```python
from build123d import *

# Parameters (mm, degrees)
F1_DEPTH = 25.4
F3_D     = 12.7
F4_D     = 12.7
F5_R     = 5.08


with BuildPart() as f1:
    # F0 (on Front) → F1 (new body)
    with BuildSketch(Plane.XZ):
        with BuildLine():
            Line((-25.4, 19.05), (-50.8, 19.05))
            Line((-50.8, 19.05), (-50.8, -19.05))
            Line((-50.8, -19.05), (50.8, -19.05))
            Line((50.8, -19.05), (50.8, 19.05))
            Line((50.8, 19.05), (25.4, 19.05))
            ThreePointArc((25.4, 19.05), (0, -6.35), (-25.4, 19.05))
        make_face()
    extrude(amount=F1_DEPTH)

    # F3 (through all)
    with Locations(Plane.XY.offset(19.05)):
        with Locations((-38.1, -12.7)):
            Hole(F3_D / 2)

    # F4 (through all)
    with Locations(Plane.XY.offset(19.05)):
        with Locations((38.1, -12.7)):
            Hole(F4_D / 2)

    # F5
    f5_edges = [f1.edges().sort_by_distance(p)[0] for p in [
        (50.8, 0, 0),
        (-50.8, 0, 0),
        (0, 0, -19.05),
        (-50.8, -12.7, -19.05),
        (-50.8, -12.7, 19.05),
        (-50.8, -25.4, 0),
        (0, -25.4, -19.05),
        (50.8, -25.4, 0),
    ]]
    fillet(f5_edges, radius=F5_R)


solid = f1.part
```
The listing builds one solid part. Answer for the finished solid, in the listing's coordinates (mm). Give positions to 0.01 mm unless a question says otherwise; leave off trailing zeros. Order: outer loops, then holes, each group sorted by start corner. A loop starts at its lowest first (then second) coordinate and runs counter-clockwise, first axis right, second up. Notation, with made-up numbers: (35, -5.5) -> (93, -5.5) arc R29 ccw to (93, 22.5) -> close; hole circle Ø10 at (54, 28.5). An arc over 180 degrees is marked (long way). One line per item, written item: value.
1) A flat-ended cylindrical pin translates along its axis: P1, Ø3, axis at x = 3.5, y = -11.5, coming from the +Z side. Find the tip coordinate at first contact, or state that the pin passes through.
Reported:
P1: stops at z = -5.85
2) Determine the mould class of faces 1 (the cylindrical face through (32.234, -15.132, -0.267)), 2 (the flat face through (-50.8, -13, 0)), 3 (the cylindrical face through (-31.756, -12.421, -0.267)), 4 (the flat face through (2, -13, -19.05)) for opening direction X: pulls with the +X half, pulls with the -X half, needs draft (parallel to the pull), parting line crosses it, or undercut.
Reported:
face 1: undercut
face 2: pulls with the -X half
face 3: undercut
face 4: needs draft
3) Find section B-B, the plane y = -12.7. Determine the outline of the cut face in (x, z).
Reported:
outline: (-50.8, -13.97) arc R5.08 ccw to (-45.72, -19.05) -> (-44.45, -19.05) -> (-44.45, 19.05) -> (-45.72, 19.05) arc R5.08 ccw to (-50.8, 13.97) -> close; (-31.75, -19.05) -> (31.75, -19.05) -> (31.75, 19.05) -> (25.4, 19.05) arc R25.4 cw to (-25.4, 19.05) -> (-31.75, 19.05) -> close; (44.45, -19.05) -> (50.8, -19.05) -> (50.8, 19.05) -> (44.45, 19.05) -> close
4) Find section D-D, the plane z = 15.5. Determine the outline of the cut face in (x, y).
Reported:
outline: (-50.56, -21.85) arc R5.08 ccw to (-45.72, -25.4) -> (-25.15, -25.4) -> (-25.15, 0) -> (-45.72, 0) arc R5.08 ccw to (-50.56, -3.55) -> close; (25.15, -25.4) -> (45.72, -25.4) arc R5.08 ccw to (50.8, -20.32) -> (50.8, -5.08) arc R5.08 ccw to (45.72, 0) -> (25.15, 0) -> close; hole circle Ø12.7 at (-38.1, -12.7); hole circle Ø12.7 at (38.1, -12.7)
5) Find section C-C, the plane z = 9. Determine the outline of the cut face in (x, y).
Reported:
outline: (-50.8, -20.32) arc R5.08 ccw to (-45.72, -25.4) -> (-23.33, -25.4) -> (-23.33, 0) -> (-45.72, 0) arc R5.08 ccw to (-50.8, -5.08) -> close; (23.33, -25.4) -> (45.72, -25.4) arc R5.08 ccw to (50.8, -20.32) -> (50.8, -5.08) arc R5.08 ccw to (45.72, 0) -> (23.33, 0) -> close; hole circle Ø12.7 at (-38.1, -12.7); hole circle Ø12.7 at (38.1, -12.7)
6) Find section A-A, the plane x = 38.1. Determine the outline of the cut face in (y, z), plus the area to 3 significant figures.
Reported:
outline: (-25.4, -13.97) arc R5.08 ccw to (-20.32, -19.05) -> (-19.05, -19.05) -> (-19.05, 19.05) -> (-25.4, 19.05) -> close; (-6.35, -19.05) -> (-5.08, -19.05) arc R5.08 ccw to (0, -13.97) -> (0, 19.05) -> (-6.35, 19.05) -> close
area: 473 mm^2
7) Find the intervals of material crossed by line 1 (Y direction, x = -38, z = -3); line 2 (X direction, y = -10, z = 9); line 3 (X direction, y = -11, z = 13.5), in increasing order.
Reported:
line 1: y = -25.4 to -19.05, -6.35 to 0
line 2: x = -50.8 to -43.85, -32.35 to -23.33, 23.33 to 32.35, 43.85 to 50.8
line 3: x = -50.8 to -44.22, -31.98 to -24.79, 24.79 to 31.98, 44.22 to 50.8
